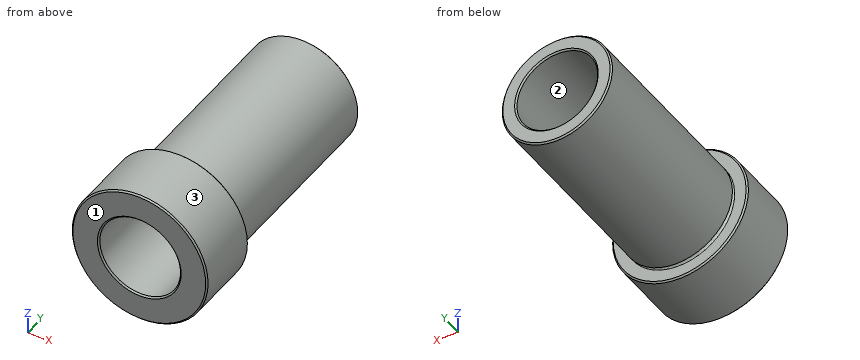
from build123d import *

# Parameters (mm, degrees)
SKIZZE1_R                       = 9.25
AUFSATZ_LINEAR_AUSTRAGEN1_DEPTH = 9
SKIZZE2_R                       = 7.5
AUFSATZ_LINEAR_AUSTRAGEN2_DEPTH = 27
SKIZZE3_R                       = 5.5
SCHNITT_LINEAR_AUSTRAGEN1_DEPTH = 40
FASE1_SIZE                      = 0.2
SKIZZE4_R                       = 0.25


with BuildPart() as part:
    # Skizze1 → Aufsatz-Linear austragen1 (new body)
    with BuildSketch(Plane(origin=(0, 0, 0), x_dir=(1, 0, 0), z_dir=(0, 1, 0))):
        Circle(SKIZZE1_R)
    extrude(amount=AUFSATZ_LINEAR_AUSTRAGEN1_DEPTH)

    # Skizze2 → Aufsatz-Linear austragen2 (add)
    with BuildSketch(Plane(origin=(0, 9, 0), x_dir=(1, 0, 0), z_dir=(0, 1, 0))):
        Circle(SKIZZE2_R)
    extrude(amount=AUFSATZ_LINEAR_AUSTRAGEN2_DEPTH)

    # Skizze3 → Schnitt-Linear austragen1 (cut)
    with BuildSketch(Plane.XZ):
        Circle(SKIZZE3_R)
    extrude(amount=-SCHNITT_LINEAR_AUSTRAGEN1_DEPTH, mode=Mode.SUBTRACT)

    # Fase1
    fase1_edges = [part.edges().sort_by_distance(p)[0] for p in [
        (-5.5, 36, 0),
        (-5.5, 0, 0),
        (-9.25, 0, 0),
        (-9.25, 9, 0),
        (-7.5, 36, 0),
    ]]
    chamfer(fase1_edges, length=FASE1_SIZE)

    # Skizze4 → Schnitt-Rotation1 (revolve, cut)
    with BuildSketch(Plane(origin=(0, 0, 0), x_dir=(0, 0, -1), z_dir=(1, 0, 0))):
        with Locations((-7.5, 9.25)):
            Circle(SKIZZE4_R)
    revolve(axis=Axis((0, 12.492787288, 0), (0, -1, 0)), mode=Mode.SUBTRACT)


solid = part.part
Design review of the part built by this model. Coordinates are the model's own, in mm. Face numbers are marked on the shaded views. Round coordinates to 2 decimals unless told otherwise and drop trailing zeros. Order: outer loops, then holes, each group sorted by start corner. A loop starts at its lowest first (then second) coordinate and runs counter-clockwise, first axis right, second up.
1) For L1, parallel to Z at x = 0, y = 17.5; L2, parallel to Y at x = 4.25, z = -8; L3, parallel to Z at x = -3, y = 12.5, list the stretches that pass through material, from the lowest coordinate up.
The answers:
L1: z = -7.5 to -5.5, 5.5 to 7.5
L2: y = 0.01 to 8.99
L3: z = -6.87 to -4.61, 4.61 to 6.87
2) Clearance check with flat-ended pins moving along their axes: pin 1 Ø1 at (x, y) = (-4.5, 4.5) entering from +Z; pin 2 Ø6 at (y, z) = (26, 4.5) entering from +X; pin 3 Ø4 at (y, z) = (20, 6) entering from +X. State where each tip first meets the part, or that it passes through.
The answers:
pin 1: stops at z = 8.34
pin 2: stops at x = 7.35
pin 3: stops at x = 6.34
3) Consider section C-C (y = 12). State the section outline as (x, z) points.
The answers:
outline: circle Ø15 at (0, 0); hole circle Ø11 at (0, 0)
4) Consider section A-A (z = 0). State the section outline as (x, y) points, plus the area to 3 significant figures.
The answers:
outline: (-9.25, 0.2) - (-9.05, 0) - (-5.7, 0) - (-5.5, 0.2) - (-5.5, 35.8) - (-5.7, 36) - (-7.3, 36) - (-7.5, 35.8) - (-7.5, 9.5) arc R0.25 cw to (-7.5, 9) - (-9.05, 9) - (-9.25, 8.8) - close; (5.5, 0.2) - (5.7, 0) - (9.05, 0) - (9.25, 0.2) - (9.25, 8.8) - (9.05, 9) - (7.5, 9) arc R0.25 cw to (7.5, 9.5) - (7.5, 35.8) - (7.3, 36) - (5.7, 36) - (5.5, 35.8) - close
area: 175 mm2
5) Consider section B-B (x = 0). State the section outline as (y, z) points.
The answers:
outline: (0, -9.05) - (0.2, -9.25) - (8.8, -9.25) - (9, -9.05) - (9, -7.5) arc R0.25 cw to (9.5, -7.5) - (35.8, -7.5) - (36, -7.3) - (36, -5.7) - (35.8, -5.5) - (0.2, -5.5) - (0, -5.7) - close; (0, 5.7) - (0.2, 5.5) - (35.8, 5.5) - (36, 5.7) - (36, 7.3) - (35.8, 7.5) - (9.5, 7.5) arc R0.25 cw to (9, 7.5) - (9, 9.05) - (8.8, 9.25) - (0.2, 9.25) - (0, 9.05) - close
6) Draft analysis for pull direction Z (two halves, no side actions). For the marked faces 1, 2 and 3, state which applies: released by +Z, released by -Z, zero draft, split by the parting line, or undercut.
The answers:
face 1: zero draft
face 2: undercut
face 3: split by the parting line
